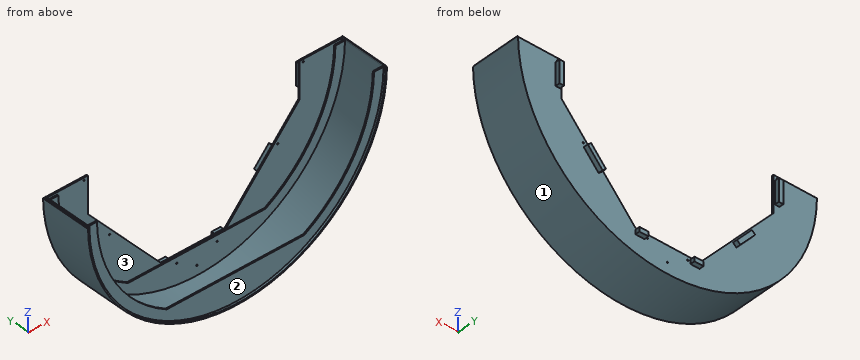
```python
from build123d import *

# Parameters (mm, degrees)
BOSS_EXTRUDE2_DEPTH      = 3
BOSS_EXTRUDE2_DEPTH_BACK = 109.6
SKETCH3_R                = 333
SKETCH3_R_2              = 330
SKETCH5_R                = 330
BOSS_EXTRUDE4_DEPTH      = 3
SKETCH6_R                = 333
BOSS_EXTRUDE6_DEPTH      = 3
SKETCH17_R               = 330
BOSS_EXTRUDE9_DEPTH      = 3
CUT_EXTRUDE1_DEPTH       = 503.240857237
CUT_EXTRUDE1_DEPTH_BACK  = 503.240857237
SKETCH18_W               = 721.551246538
SKETCH18_H               = 348.822819085
SKETCH19_W               = 10
SKETCH19_H               = 50
SKETCH19_W_2             = 20
SKETCH19_H_2             = 10
BOSS_EXTRUDE10_DEPTH     = 10
SKETCH23_W               = 1.500186503
SKETCH23_H               = 109.4
BOSS_EXTRUDE11_DEPTH     = 4
CUT_EXTRUDE2_START       = -11
SKETCH25_R               = 1.5
CUT_EXTRUDE2_DEPTH       = 11


with BuildPart() as part:
    # Sketch3 → Boss-Extrude2 (new, two sides: drawn at the far end of the back side and taken through both)
    with BuildSketch(Plane(origin=(0, 0, 0), x_dir=(1, 0, 0), z_dir=(0, 1, 0)).offset(-BOSS_EXTRUDE2_DEPTH_BACK)):
        with Locations(Location((-11.008302555, 15.174390861, 0), (0, 0, 270))):
            Circle(SKETCH3_R)
        with Locations(Location((-11.008302555, 15.174390861, 0), (0, 0, 270))):
            Circle(SKETCH3_R_2, mode=Mode.SUBTRACT)
    extrude(amount=BOSS_EXTRUDE2_DEPTH + BOSS_EXTRUDE2_DEPTH_BACK)

    # Sketch5 → Boss-Extrude4 (add)
    with BuildSketch(Plane.XZ.offset(104.6)):
        with Locations(Location((-11.008302555, -15.174390861, 0), (0, 0, 90))):
            Circle(SKETCH5_R)
        with BuildLine():
            Line((-164.332788108, -283.060090014), (142.316182998, -283.060090014))
            ThreePointArc((142.316182998, -283.060090014), (-11.008302555, 293.485852256), (-164.332788108, -283.060090014))
        make_face(mode=Mode.SUBTRACT)
    extrude(amount=-BOSS_EXTRUDE4_DEPTH)

    # Sketch6 → Boss-Extrude6 (add)
    with BuildSketch(Plane(origin=(0, 0, 0), x_dir=(1, 0, 0), z_dir=(0, 1, 0))):
        with Locations(Location((-11.008302555, 15.174390861, 0), (0, 0, 270))):
            Circle(SKETCH6_R)
        Polygon((187.991697445, -189.598621739), (187.991697445, 20.401378261), (224.991697445, 20.401378261), (224.991697445, 100.970480915), (60.317326344, 288.174390861), (-82.333931455, 288.174390861), (-247.008302555, 100.970480915), (-247.008302555, 20.401378261), (-210.008302555, 20.401378261), (-210.008302555, -189.598621739), align=None, mode=Mode.SUBTRACT)
    extrude(amount=BOSS_EXTRUDE6_DEPTH)

    # Sketch17 → Boss-Extrude9 (add)
    with BuildSketch(Plane(origin=(0, -5, 0), x_dir=(1, 0, 0), z_dir=(0, 1, 0))):
        with Locations(Location((-11.008302555, 15.174390861, 0), (0, 0, 270))):
            Circle(SKETCH17_R)
        with BuildLine():
            Line((142.316182998, 283.060090014), (-164.332788108, 283.060090014))
            ThreePointArc((-164.332788108, 283.060090014), (-11.008302555, -293.485852256), (142.316182998, 283.060090014))
        make_face(mode=Mode.SUBTRACT)
    extrude(amount=-BOSS_EXTRUDE9_DEPTH)

    # Sketch18 → Cut-Extrude1 (cut, two sides: drawn at the far end of the back side and taken through both)
    with BuildSketch(Plane(origin=(0, 3, 0), x_dir=(1, 0, 0), z_dir=(0, 1, 0)).offset(-CUT_EXTRUDE1_DEPTH_BACK)):
        with Locations((-2.663832357, -154.010031282)):
            Rectangle(SKETCH18_W, SKETCH18_H)
    extrude(amount=CUT_EXTRUDE1_DEPTH + CUT_EXTRUDE1_DEPTH_BACK, mode=Mode.SUBTRACT)

    # Sketch19 → Boss-Extrude10 (add)
    with BuildSketch(Plane(origin=(0, 3, 0), x_dir=(1, 0, 0), z_dir=(0, 1, 0))):
        Polygon((-190.005313879, 170.617155509), (-156.981273896, 208.159302266), (-164.489703247, 214.764110263), (-197.513743231, 177.221963505), align=None)
        Polygon((167.988708769, 170.617155509), (134.964668786, 208.159302266), (142.473098137, 214.764110263), (175.49713812, 177.221963505), align=None)
        with Locations((-255.208302555, 56.010036487)):
            Rectangle(SKETCH19_W, SKETCH19_H)
        with Locations((233.191697445, 56.010036487)):
            Rectangle(SKETCH19_W, SKETCH19_H)
        with Locations((-72.333931455, 296.374390861)):
            Rectangle(SKETCH19_W_2, SKETCH19_H_2)
        with Locations((50.317326344, 296.374390861)):
            Rectangle(SKETCH19_W_2, SKETCH19_H_2)
    extrude(amount=BOSS_EXTRUDE10_DEPTH)

    # Sketch23 → Boss-Extrude11 (add)
    with BuildSketch(Plane.XY.offset(-20.401378261)):
        with Locations((319.700392044, -54.9)):
            Rectangle(SKETCH23_W, SKETCH23_H)
        with Locations((-341.716997154, -54.9)):
            Rectangle(SKETCH23_W, SKETCH23_H)
    extrude(amount=BOSS_EXTRUDE11_DEPTH)

    # Sketch25 → Cut-Extrude2 (cut)
    with BuildSketch(Plane(origin=(0, 3, 0), x_dir=(1, 0, 0), z_dir=(0, 1, 0)).offset(CUT_EXTRUDE2_START)):
        with Locations(Location((-56.008302555, 296.667912331, 0), (0, 0, 270))):
            Circle(SKETCH25_R)
        with Locations(Location((33.991697445, 296.667912331, 0), (0, 0, 270))):
            Circle(SKETCH25_R)
        with Locations(Location((-11.008302555, 323.834633978, 0), (0, 0, 270))):
            Circle(SKETCH25_R)
        with Locations(Location((-198.376364015, 168.671082504, 0), (0, 0, 270))):
            Circle(SKETCH25_R)
        with Locations(Location((176.359758905, 168.671082504, 0), (0, 0, 270))):
            Circle(SKETCH25_R)
        with Locations(Location((-255.208302555, 25.978544832, 0), (0, 0, 270))):
            Circle(SKETCH25_R)
        with Locations(Location((233.191697445, 25.978544832, 0), (0, 0, 270))):
            Circle(SKETCH25_R)
    extrude(amount=CUT_EXTRUDE2_DEPTH, mode=Mode.SUBTRACT)


solid = part.part
```
Geometry: final body of the model. Coordinates: model frame, mm. Face numbers are marked on the shaded views. Round coordinates to 2 decimals unless told otherwise and drop trailing zeros. Order: outer loops, then holes, each group sorted by start corner. A loop starts at its lowest first (then second) coordinate and runs counter-clockwise, first axis right, second up. Notation, with made-up numbers: (72, -17.5) - (105, -17.5) arc R34 cw to (105, 14.5) - close; hole circle Ø1 at (66, -34.5). An arc over 180 degrees is marked (long way). Write item = value, one per line. Start each with the question number.
Q1. Pull-direction query (Y, two-part tool) for the marked faces 1, 2 and 3; classes: +Y half, -Y half, draft (parallel to the pull), parting line (faces both ways), or undercut.
Q2. Ray query, line 1 (Y direction, x = 86, z = -326); line 2 (X direction, y = -55, z = -103); line 3 (X direction, y = -1.5, z = -126). Return the intervals inside material, ascending. Write a range as from..to.
Q3. Cut plane C-C on x = -214. Return the cut outline in (y, z), and give its area (3 significant figures).
Q4. Cut plane A-A on y = -46.5. Return the cut outline in (x, z), and give its area (3 significant figures).
Q5. Cut plane B-B on z = -262. Return the cut outline in (x, y), and give its area (3 significant figures).
Q6. Pin query (flat end, axial travel): pin 1 (2.5 mm diameter, centred on x = -198.38, z = -168.67, fed in from +Y); pin 2 (12 mm diameter, centred on x = -71.5, y = -11, fed in from -Z); pin 3 (12 mm diameter, centred on y = -76.5, z = -166, fed in from +X); pin 4 (2.5 mm diameter, centred on x = 308.5, y = -103.5, fed in from +Z). Return the tip coordinate at first contact, or that it passes through.
Outcome:
q1.face_1 = draft
q1.face_2 = -Y half
q1.face_3 = undercut
q2.line_1 = -104.6..-101.6, -8..-5, 0..3
q2.line_2 = -332.22..-329.11, 307.09..310.2
q2.line_3 = -325.03..-321.84, 299.83..303.01
q3.outline = (-109.6, -279.15) - (3, -279.15) - (3, -138.49) - (0, -138.49) - (0, -275.36) - (-5, -275.36) - (-5, -247.69) - (-8, -247.69) - (-8, -275.36) - (-101.6, -275.36) - (-101.6, -247.69) - (-104.6, -247.69) - (-104.6, -275.36) - (-109.6, -275.36) - close
q3.area = 1,000 mm^2
q4.outline = (-343.97, -20.4) arc R333 ccw to (321.95, -20.4) - (320.45, -20.4) - (320.45, -16.4) - (318.95, -16.4) - (318.95, -20.4) arc R330 cw to (-340.97, -20.4) - (-340.97, -16.4) - (-342.47, -16.4) - (-342.47, -20.4) - close
q4.area = 3,100 mm^2
q5.outline = (-234.54, -109.6) - (-230.05, -109.6) - (-230.05, -104.6) - (-196.34, -104.6) - (-196.34, -101.6) - (-230.05, -101.6) - (-230.05, -8) - (-196.34, -8) - (-196.34, -5) - (-230.05, -5) - (-230.05, 0) - (-105.36, 0) - (-105.36, 3) - (-234.54, 3) - close; (83.34, 0) - (208.03, 0) - (208.03, -5) - (174.32, -5) - (174.32, -8) - (208.03, -8) - (208.03, -101.6) - (174.32, -101.6) - (174.32, -104.6) - (208.03, -104.6) - (208.03, -109.6) - (212.52, -109.6) - (212.52, 3) - (83.34, 3) - close
q5.area = 2,160 mm^2
q6.pin_1 = through
q6.pin_2 = -343.69
q6.pin_3 = 288.85
q6.pin_4 = -20.4
